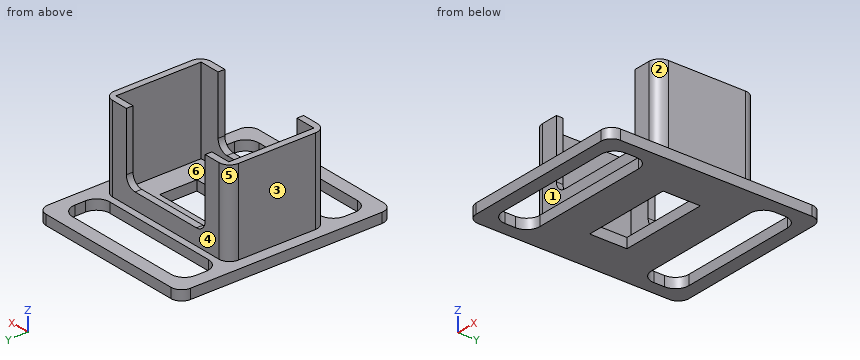
from build123d import *

# Parameters (mm, degrees)
F0_W      = 82.55
F0_H      = 101.6
F1_DEPTH  = 4.7625
F2_W      = 71.755
F2_H      = 46.99
F2_W_2    = 65.405
F2_H_2    = 40.64
F3_DEPTH  = 40.64
F4_W      = 45.72
F4_H      = 32.9846274108
F5_DEPTH  = 40.132
F6_R      = 5.08
F7_R      = 5.08
F9_DEPTH  = 25.4
F10_W     = 42.545
F10_H     = 17.78
F11_DEPTH = 25.4


with BuildPart() as f1:
    # F0 (on Top) → F1 (new body)
    with BuildSketch(Plane.XY):
        Rectangle(F0_W, F0_H)
    extrude(amount=F1_DEPTH)

    # F2 (on face) → F3 (join)
    with BuildSketch(Plane.XY.offset(4.7625)):
        Rectangle(F2_W, F2_H)
        Rectangle(F2_W_2, F2_H_2, mode=Mode.SUBTRACT)
    extrude(amount=F3_DEPTH)

    # F4 (on Front) → F5 (cut, symmetric)
    with BuildSketch(Plane.XZ):
        with Locations((0, 28.9101862946)):
            Rectangle(F4_W, F4_H)
    extrude(amount=F5_DEPTH, both=True, mode=Mode.SUBTRACT)

    # F6
    f6_edges = [f1.edges().sort_by_distance(p)[0] for p in [
        (-22.86, 21.9075, 12.417873),
        (-22.86, -21.9075, 12.417873),
        (22.86, 21.9075, 12.417873),
        (22.86, -21.9075, 12.417873),
    ]]
    fillet(f6_edges, radius=F6_R)

    # F7
    f7_edges = [f1.edges().sort_by_distance(p)[0] for p in [
        (-35.8775, -23.495, 25.0825),
        (-35.8775, 23.495, 25.0825),
        (35.8775, -23.495, 25.0825),
        (35.8775, 23.495, 25.0825),
        (-41.275, -50.8, 2.38125),
        (41.275, -50.8, 2.38125),
        (41.275, 50.8, 2.38125),
        (-41.275, 50.8, 2.38125),
    ]]
    fillet(f7_edges, radius=F7_R)

    # F8 (on face) → F9 (cut)
    with BuildSketch(Plane.XY.offset(4.7625)):
        with BuildLine():
            Line((28.575, 44.45), (-28.575, 44.45))
            ThreePointArc((-28.575, 44.45), (-33.0651280605, 42.5901280605), (-34.925, 38.1))
            Line((-34.925, 38.1), (-34.925, 33.02))
            ThreePointArc((-34.925, 33.02), (-33.0651280605, 28.5298719395), (-28.575, 26.67))
            Line((-28.575, 26.67), (28.575, 26.67))
            ThreePointArc((28.575, 26.67), (33.0651280605, 28.5298719395), (34.925, 33.02))
            Line((34.925, 33.02), (34.925, 38.1))
            ThreePointArc((34.925, 38.1), (33.0651280605, 42.5901280605), (28.575, 44.45))
        make_face()
        with BuildLine():
            Line((28.575, -26.67), (-28.575, -26.67))
            ThreePointArc((-28.575, -26.67), (-33.0651280605, -28.5298719395), (-34.925, -33.02))
            Line((-34.925, -33.02), (-34.925, -38.1))
            ThreePointArc((-34.925, -38.1), (-33.0651280605, -42.5901280605), (-28.575, -44.45))
            Line((-28.575, -44.45), (28.575, -44.45))
            ThreePointArc((28.575, -44.45), (33.0651280605, -42.5901280605), (34.925, -38.1))
            Line((34.925, -38.1), (34.925, -33.02))
            ThreePointArc((34.925, -33.02), (33.0651280605, -28.5298719395), (28.575, -26.67))
        make_face()
    extrude(amount=-F9_DEPTH, mode=Mode.SUBTRACT)

    # F10 (on face) → F11 (cut)
    with BuildSketch(Plane.XY.offset(4.7625)):
        Rectangle(F10_W, F10_H)
    extrude(amount=-F11_DEPTH, mode=Mode.SUBTRACT)


solid = f1.part
Check sheet for the modelled part. Datum: model origin and axes. Units: mm. Face numbers are marked on the shaded views. A direction names the side the tool comes from. Give positions to 0.01 mm unless a question says otherwise; leave off trailing zeros. Loops run counter-clockwise (first coordinate to the right, second up) from the corner with the lowest first, then second, coordinate; pieces in that order, holes last. Notation, with made-up numbers: M -35.5,18 L -17.5,18 A14 ccw -17.5,28 Z; hole C 74,66 d1. An arc over 180 degrees is marked long. Use a Markdown table: item, result. Add a question column.
Q1. Sectioned sample at C-C, the plane y = 13.5. Record the cut outline in (x, z) (1 decimal).
Q2. Go/stop test with flat-tipped pins: pin 1 (3 mm diameter, centred on y = 2.5, z = 36, fed in from +X); pin 2 (12 mm diameter, centred on x = -2, z = 16.5, fed in from -Y) (3 decimals); pin 3 (3.5 mm diameter, centred on x = 7, y = -22, fed in from +Z). Record where each tip stops, or that it passes through.
Q3. Sectioned sample at A-A, the plane x = -4. Give the number of separate pieces and of enclosed holes in the cut face, then the cut area to 3 significant figures.
Q4. Tool access check on the marked faces 1, 2 and 3. Record the directions out of +Z, -Z, +X, -X, +Y, -Y that give a thin tool (end or side, any length) a straight path to the whole face; none if there is none.
Q5. Scan lines: line 1 along X through (y, z) = (-6.5, 9); line 2 along Y through (x, z) = (-2.5, 4); line 3 along X through (y, z) = (4, 4) (1 decimal). Record each from-to range of solid material in increasing order. Write a range as [from, to].
Q6. Sectioned sample at B-B, the plane z = 23. Record the cut outline in (x, y) (1 decimal).
Q7. Mould release check, pull along X, two halves, no side actions. Record for the marked faces 4, 5 and 6: pulls with the +X half, pulls with the -X half, needs draft (parallel to the pull), parting line crosses it, or undercut.
Q8. Sectioned sample at D-D, the plane z = 6.5. Record the cut outline in (x, y) (1 decimal).
Verdict:
| question | item | result |
|---|---|---|
| 1 | outline | M -41.3,0 L 41.3,0 L 41.3,4.8 L 35.9,4.8 L 35.9,45.4 L 32.7,45.4 L 32.7,4.8 L -32.7,4.8 L -32.7,45.4 L -35.9,45.4 L -35.9,4.8 L -41.3,4.8 Z |
| 2 | pin 1 | x = 35.88 |
| 2 | pin 2 | y = -23.495 |
| 2 | pin 3 | z = 12.42 |
| 3 | separate pieces | 4 |
| 3 | enclosed holes | 0 |
| 3 | area | 278 mm^2 |
| 4 | face 1 | +Z, +X, -X, -Y |
| 4 | face 2 | +Z, +X, -Y |
| 4 | face 3 | +Z, -X, +Y, -Y |
| 5 | line 1 | [-35.88, -32.7], [32.7, 35.88] |
| 5 | line 2 | [-50.8, -44.45], [-26.67, -8.89], [8.89, 26.67], [44.45, 50.8] |
| 5 | line 3 | [-41.3, -21.3], [21.3, 41.3] |
| 6 | outline | M -35.9,-18.4 A5.1 ccw -30.8,-23.5 L -22.9,-23.5 L -22.9,-20.3 L -32.7,-20.3 L -32.7,20.3 L -22.9,20.3 L -22.9,23.5 L -30.8,23.5 A5.1 ccw -35.9,18.4 Z; M 22.9,-23.5 L 30.8,-23.5 A5.1 ccw 35.9,-18.4 L 35.9,18.4 A5.1 ccw 30.8,23.5 L 22.9,23.5 L 22.9,20.3 L 32.7,20.3 L 32.7,-20.3 L 22.9,-20.3 Z |
| 7 | face 4 | needs draft |
| 7 | face 5 | pulls with the -X half |
| 7 | face 6 | undercut |
| 8 | outline | M -35.9,-18.4 A5.1 ccw -30.8,-23.5 L 30.8,-23.5 A5.1 ccw 35.9,-18.4 L 35.9,18.4 A5.1 ccw 30.8,23.5 L -30.8,23.5 A5.1 ccw -35.9,18.4 Z; hole M -32.7,-20.3 L 32.7,-20.3 L 32.7,20.3 L -32.7,20.3 Z |
